The listing builds one solid part. Answer for the finished solid, in the listing's coordinates (mm). A direction names the side the tool comes from. Coordinates: 2 decimals unless noted, no trailing zeros. Order: outer loops, then holes, each group sorted by start corner. A loop starts at its lowest first (then second) coordinate and runs counter-clockwise, first axis right, second up. Notation, with made-up numbers: (-24.75, -9) -> (-18.75, -9) arc R26 ccw to (-18.75, 23) -> close; hole circle Ø7 at (46, -10). An arc over 180 degrees is marked (long way). Write item = value, one per line. Start each with the question number.
```python
from build123d import *

# Parameters (mm, degrees)
SKETCH1_R           = 1.5
SKETCH1_W           = 5
SKETCH1_H           = 3
BOSS_EXTRUDE1_DEPTH = 3


with BuildPart() as part:
    # Sketch1 → Boss-Extrude1 (new body)
    with BuildSketch(Plane(origin=(0, 0, 0), x_dir=(1, 0, 0), z_dir=(0, 1, 0))):
        with BuildLine():
            Line((0, 0), (-60, 0))
            ThreePointArc((-60, 0), (-65, 5), (-60, 10))
            Line((-60, 10), (0, 10))
            ThreePointArc((0, 10), (5, 5), (0, 0))
        make_face()
        with Locations((-60, 5)):
            Circle(SKETCH1_R, mode=Mode.SUBTRACT)
        with Locations((-40, 5)):
            Circle(SKETCH1_R, mode=Mode.SUBTRACT)
        with Locations((-2.5, 2.5)):
            Rectangle(SKETCH1_W, SKETCH1_H, mode=Mode.SUBTRACT)
        with Locations((-2.5, 7.5)):
            Rectangle(SKETCH1_W, SKETCH1_H, mode=Mode.SUBTRACT)
    extrude(amount=BOSS_EXTRUDE1_DEPTH)


solid = part.part
```
Item 1: Section B-B, the plane y = 1.2 is taken. Give the vertices of the cut face in (x, z), then the cut area to 3 significant figures.
Item 2: For a pull along X with two mould halves and no side action, classify faces 3 (the flat face through (-30, 1, -10)), 4 (the cylindrical face through (5, 1, -5)), 5 (the flat face through (-3, 1, -1)), 6 (the flat face through (-3, 1, -4)) as pulls with the +X half, pulls with the -X half, needs draft (parallel to the pull), parting line crosses it, or undercut.
Item 3: Which of the six approach directions +Z, -Z, +X, -X, +Y, -Y give full straight-line access (tool end or side, diameter ignored) to faces 1 (the flat face through (-30, 0, -5)), 2 (the flat face through (-5, 1, -7))?
Item 4: Section C-C, the plane z = -5 is taken. Give the vertices of the cut face in (x, y).
Item 5: Consider probe 1 along X at (y, z) = (1.7, -5); probe 2 along Z at (x, y) = (-40, 1.3); probe 3 along Z at (x, y) = (-61, 0.45). Determine where each line is inside the solid, lowest interval first.
Item 6: Section A-A, the plane x = -40 is taken. Give the vertices of the cut face in (y, z), then the cut area to 3 significant figures.
Item 7: Each of these flat-tipped pins is pushed along its axis until it touches: pin 1 (1 mm diameter, centred on y = 1, z = -2.5, fed in from -X); pin 2 (1 mm diameter, centred on y = 0.5, z = -6, fed in from +X); pin 3 (1.5 mm diameter, centred on y = 1, z = -8, fed in from -X). Where does it stop, or does it pass through?
A:
q1.outline = (-60, -10) -> (0, -10) arc R5 ccw to (0, 0) -> (-60, 0) arc R5 ccw to start; hole circle Ø3 at (-60, -5); hole circle Ø3 at (-40, -5); hole (-5, -9) -> (0, -9) -> (0, -6) -> (-5, -6) -> close; hole (-5, -4) -> (0, -4) -> (0, -1) -> (-5, -1) -> close
q1.area = 634 mm^2
q2.face_3 = needs draft
q2.face_4 = pulls with the +X half
q2.face_5 = undercut
q2.face_6 = undercut
q3.face_1 = +Z, -Z, +X, -X, -Y
q3.face_2 = +Y, -Y
q4.outline = (-65, 0) -> (-61.5, 0) -> (-61.5, 3) -> (-65, 3) -> close; (-58.5, 0) -> (-41.5, 0) -> (-41.5, 3) -> (-58.5, 3) -> close; (-38.5, 0) -> (5, 0) -> (5, 3) -> (-38.5, 3) -> close
q5.probe_1 = -65 to -61.5, -58.5 to -41.5, -38.5 to 5
q5.probe_2 = -10 to -6.5, -3.5 to 0
q5.probe_3 = -9.9 to -6.12, -3.88 to -0.1
q6.outline = (0, -10) -> (3, -10) -> (3, -6.5) -> (0, -6.5) -> close; (0, -3.5) -> (3, -3.5) -> (3, 0) -> (0, 0) -> close
q6.area = 21.0 mm^2
q7.pin_1 = -64.58
q7.pin_2 = 4.97
q7.pin_3 = -64.47
